Verification items for the finished model (mm, model axes). Coordinates: 2 decimals unless noted, no trailing zeros. Order: outer loops, then holes, each group sorted by start corner. A loop starts at its lowest first (then second) coordinate and runs counter-clockwise, first axis right, second up.
Q1. Cross-section at C-C, the plane z = 1.65. Record the boundary of the cut face in (x, y).
Q2. Cross-section at A-A, the plane x = 79. Record the boundary of the cut face in (y, z), and give its area (3 significant figures).
Q3. Draft check along X on faces 1 (the cylindrical face through (71.908, 12.327, 1.014)), 2 (the flat face through (110.028, -2.398, 0.986)), 3 (the cylindrical face through (101.908, 0.601, 1.014)), 4 (the cylindrical face through (-7.895, -59.478, 0.986)). Enter one of: pulls with the +X half, pulls with the -X half, needs draft (parallel to the pull), parting line crosses it, or undercut.
Q4. Cross-section at B-B, the plane y = 45. Record the boundary of the cut face in (x, z).
Q5. Cross-section at D-D, the plane x = 55. Record the boundary of the cut face in (y, z).
Q6. Depth check by flat-ended pin: P1, Ø0.6, axis at x = 75.5, z = 0.5, coming from the -Y side. Enter the tip coordinate at first touch or a pass-through.
Q7. Thickness scan on line 1 (Y direction, x = 100, z = 0.45); line 2 (Y direction, x = 70, z = 0.9); line 3 (Y direction, x = 66.5, z = 1.4). Record the ranges inside material, lowest first.
from build123d import *

# Parameters (mm, degrees)
SKETCH1_R           = 7.5
SKETCH1_R_2         = 25
BOSS_EXTRUDE1_DEPTH = 2
CUT_EXTRUDE1_REACH  = 145.192
SKETCH2_R           = 2
SKETCH3_R           = 2
CUT_EXTRUDE2_DEPTH  = 10


with BuildPart() as part:
    # Sketch1 → Boss-Extrude1 (new body)
    # profile 1 of 2: a face of its own
    with BuildSketch(Plane.XY):
        with BuildLine():
            ThreePointArc((-60, 0), (-52.867640737, 28.372743309), (-33.166247904, 50))
            Line((-33.166247904, 50), (-60, 50))
            Line((-60, 50), (-60, 0))
        make_face()
    # profile 2 of 2: a face of its own
    with BuildSketch(Plane.XY):
        with BuildLine():
            ThreePointArc((0, 60), (-17.320508076, 57.445626465), (-33.166247904, 50))
            ThreePointArc((-33.166247904, 50), (-52.867640737, 28.372743309), (-60, 0))
            ThreePointArc((-60, 0), (-6.678621673, -59.627141576), (58.513200418, -13.274237334))
            Line((58.513200418, -13.274237334), (99.152169538, -13.274237334))
            Line((99.152169538, -13.274237334), (121.213203436, 8.786796564))
            ThreePointArc((121.213203436, 8.786796564), (127.716385975, 41.480502971), (100, 60))
            Line((100, 60), (0, 60))
        make_face()
        Circle(SKETCH1_R, mode=Mode.SUBTRACT)
        with Locations((100, 30)):
            Circle(SKETCH1_R_2, mode=Mode.SUBTRACT)
    extrude(amount=BOSS_EXTRUDE1_DEPTH)

    # Sketch2 → Cut-Extrude1 (cut, up to next)
    with BuildSketch(Plane.XY.offset(2), mode=Mode.PRIVATE) as cut_extrude1_sk1:
        with Locations((55, 45)):
            Circle(SKETCH2_R)
    cut_extrude1_tool1 = extrude(cut_extrude1_sk1.sketch, amount=-CUT_EXTRUDE1_REACH, mode=Mode.PRIVATE) & part.part
    # Sketch2 → Cut-Extrude1 (cut, up to next)
    with BuildSketch(Plane.XY.offset(2), mode=Mode.PRIVATE) as cut_extrude1_sk2:
        with Locations((70, 11.725762666)):
            Circle(SKETCH2_R)
    cut_extrude1_tool2 = extrude(cut_extrude1_sk2.sketch, amount=-CUT_EXTRUDE1_REACH, mode=Mode.PRIVATE) & part.part
    add(cut_extrude1_tool1.solids().sort_by_distance((55, 45, 2))[0], mode=Mode.SUBTRACT)
    add(cut_extrude1_tool2.solids().sort_by_distance((70, 11.725763, 2))[0], mode=Mode.SUBTRACT)

    # Sketch3 → Cut-Extrude2 (cut)
    with BuildSketch(Plane.XY.offset(2)):
        with Locations((100, 0)):
            Circle(SKETCH3_R)
    extrude(amount=-CUT_EXTRUDE2_DEPTH, mode=Mode.SUBTRACT)


solid = part.part
Check values:
1. outline: (-60, 0) arc R60 ccw to (58.51, -13.27) - (99.15, -13.27) - (121.21, 8.79) arc R30 ccw to (100, 60) - (0, 60) arc R60 ccw to (-33.17, 50) - (-60, 50) - close; hole circle Ø15 at (0, 0); hole circle Ø4 at (55, 45); hole circle Ø4 at (70, 11.73); hole circle Ø50 at (100, 30); hole circle Ø4 at (100, 0)
2. outline: (-13.27, 0) - (16.44, 0) - (16.44, 2) - (-13.27, 2) - close; (43.56, 0) - (60, 0) - (60, 2) - (43.56, 2) - close
2. area: 92.3 mm2
3. face 1: undercut
3. face 2: pulls with the +X half
3. face 3: undercut
3. face 4: parting line crosses it
4. outline: (-60, 0) - (53, 0) - (53, 2) - (-60, 2) - close; (57, 0) - (80, 0) - (80, 2) - (57, 2) - close; (120, 0) - (125.98, 0) - (125.98, 2) - (120, 2) - close
5. outline: (-23.98, 0) - (43, 0) - (43, 2) - (-23.98, 2) - close; (47, 0) - (60, 0) - (60, 2) - (47, 2) - close
6. P1: stops at y = -13.27
7. line 1: y = -12.43 to -2, 2 to 5, 55 to 60
7. line 2: y = -13.27 to 9.73, 13.73 to 60
7. line 3: y = -13.27 to 60
